Read the model definition and answer for the solid it produces. Units are mm, in the model's axes. A direction names the side the tool comes from. Round coordinates to 2 decimals unless told otherwise and drop trailing zeros. Order: outer loops, then holes, each group sorted by start corner. A loop starts at its lowest first (then second) coordinate and runs counter-clockwise, first axis right, second up. Notation, with made-up numbers: (2.25, -27) -> (17.25, -27) arc R29 ccw to (17.25, 5) -> close; hole circle Ø11 at (-19, 11). An arc over 180 degrees is marked (long way). One line per item, written item: value. Start each with the question number.
1. Section D-D (z = -27) is taken. Give the vertices of the cut face in (x, y), then the cut area to 3 significant figures.
2. The mould has two halves that part along Z. Classify faces 3 (the face through (44.014, 2.465, -24.759)), 4 (the face through (-0.565, 2.465, 50.497)), 5 (the face through (0, 3, -6)): released by +Z, released by -Z, zero draft, split by the parting line, or undercut.
3. Section A-A (x = 0) is taken. Give the vertices of the cut face in (y, z) (3 decimals).
4. Flat-ended cylindrical pins translate along their axes: pin 1 Ø1.5 at (x, z) = (28, 16) entering from -Y; pin 2 Ø1 at (x, y) = (-7, 3) entering from +Z; pin 3 Ø1.5 at (x, y) = (-1, 2.5) entering from +Z. Find the tip coordinate at first contact, or state that the pin passes through.
5. For faces 1 (the face through (-30.64, 2.54, 34.6)), 2 (the face through (39.43, 2.535, 22.706)), determine the directions among +Z, -Z, +X, -X, +Y, -Y from which every point of the face is accessible in a straight line to the end or side of a thin tool.
6. Consider line 1 (X direction, y = 4.8, z = 17.5); line 2 (X direction, y = 2.4, z = -4); line 3 (X direction, y = 3.2, z = -39.75). Determine where each line is inside the solid, lowest interval first.
7. Section C-C (z = -39.75) is taken. Give the vertices of the cut face in (x, y), then the cut area to 3 significant figures.
8. Section B-B (z = -16) is taken. Give the vertices of the cut face in (x, y).
from build123d import *

# Parameters (mm, degrees)
SKETCH1_R                = 50.5
SKETCH1_R_2              = 5.675
BOSS_EXTRUDE1_DEPTH      = 5
SKETCH4_R                = 1.7
CUT_EXTRUDE5_DEPTH       = 72.592597383
SKETCH8_R                = 1.7
CUT_EXTRUDE9_DEPTH       = 72.592597383
SKETCH9_R                = 1.7
CUT_EXTRUDE10_DEPTH      = 72.592597383
CIRPATTERN3_COUNT        = 3
CUT_EXTRUDE11_DEPTH      = 72.592597383
CIRPATTERN4_COUNT        = 3
SKETCH11_W               = 12
SKETCH11_H               = 12
CUT_EXTRUDE12_DEPTH      = 72.592597383
FILLET1_R                = 2
CUT_EXTRUDE13_DEPTH      = 72.592597383
FILLET2_R                = 10
CIRPATTERN5_COUNT        = 3
FILLET2_OF_CIRPATTERN5_R = 10


with BuildPart() as part:
    # Sketch1 → Boss-Extrude1 (new body)
    with BuildSketch(Plane(origin=(0, 0, 0), x_dir=(1, 0, 0), z_dir=(0, 1, 0))):
        with Locations(Location((0, 0, 0), (0, 0, 270))):
            Circle(SKETCH1_R)
        with Locations(Location((0, 28, 0), (0, 0, 270))):
            Circle(SKETCH1_R_2, mode=Mode.SUBTRACT)
        with Locations(Location((24.248711306, -14, 0), (0, 0, 270))):
            Circle(SKETCH1_R_2, mode=Mode.SUBTRACT)
        with Locations(Location((-24.248711306, -14, 0), (0, 0, 270))):
            Circle(SKETCH1_R_2, mode=Mode.SUBTRACT)
    extrude(amount=BOSS_EXTRUDE1_DEPTH)

    # Sketch4 → Cut-Extrude5 (cut, through all)
    with BuildSketch(Plane(origin=(0, 0, 0), x_dir=(1, 0, 0), z_dir=(0, 1, 0))):
        with Locations(Location((27.712812921, 16, 0), (0, 0, 270))):
            Circle(SKETCH4_R)
        with Locations(Location((0, -32, 0), (0, 0, 270))):
            Circle(SKETCH4_R)
        with Locations(Location((-27.712812921, 16, 0), (0, 0, 270))):
            Circle(SKETCH4_R)
    extrude(amount=CUT_EXTRUDE5_DEPTH, mode=Mode.SUBTRACT)

    # Sketch8 → Cut-Extrude9 (cut, through all)
    with BuildSketch(Plane(origin=(0, 5, 0), x_dir=(1, 0, 0), z_dir=(0, 1, 0))):
        with Locations(Location((11, 39.75, 0), (0, 0, 270))):
            Circle(SKETCH8_R)
        with Locations(Location((11, 15.75, 0), (0, 0, 270))):
            Circle(SKETCH8_R)
        with Locations(Location((-11, 39.75, 0), (0, 0, 90))):
            Circle(SKETCH8_R)
        with Locations(Location((-11, 15.75, 0), (0, 0, 90))):
            Circle(SKETCH8_R)
    cut_extrude9 = extrude(amount=-CUT_EXTRUDE9_DEPTH, mode=Mode.SUBTRACT)

    # Sketch9 → Cut-Extrude10 (cut, through all)
    with BuildSketch(Plane.XZ):
        with Locations(Location((-17.892304845, 39, 0), (0, 0, 270))):
            Circle(SKETCH9_R)
        with Locations(Location((17.892304845, 39, 0), (0, 0, 90))):
            Circle(SKETCH9_R)
    cut_extrude10 = extrude(amount=-CUT_EXTRUDE10_DEPTH, mode=Mode.SUBTRACT)

    # CirPattern3: Cut-Extrude9, Cut-Extrude10 ×3 about axis
    cirpattern3_axis = Axis((0, 0, 0), (0, 1, 0))
    add([cut_extrude9.rotate(cirpattern3_axis, i * 360 / CIRPATTERN3_COUNT) for i in range(1, CIRPATTERN3_COUNT)], mode=Mode.SUBTRACT)
    add([cut_extrude10.rotate(cirpattern3_axis, i * 360 / CIRPATTERN3_COUNT) for i in range(1, CIRPATTERN3_COUNT)], mode=Mode.SUBTRACT)

    # Sketch10 → Cut-Extrude11 (cut, through all)
    with BuildSketch(Plane(origin=(0, 5, 0), x_dir=(1, 0, 0), z_dir=(0, 1, 0))):
        with BuildLine():
            Line((-13.943212455, 41.732323521), (-15.36922282, 46.000402062))
            ThreePointArc((-15.36922282, 46.000402062), (-20.496985694, 43.955927671), (-25.359206382, 41.341996223))
            Line((-25.359206382, 41.341996223), (-23.006290326, 37.506140903))
            ThreePointArc((-23.006290326, 37.506140903), (-18.595203517, 39.87754263), (-13.943212455, 41.732323521))
        make_face()
    cut_extrude11 = extrude(amount=-CUT_EXTRUDE11_DEPTH, mode=Mode.SUBTRACT)

    # CirPattern4: Cut-Extrude11 ×3 about axis
    cirpattern4_axis = Axis((0, 0, 0), (0, 1, 0))
    for i in range(1, CIRPATTERN4_COUNT):
        add(cut_extrude11.rotate(cirpattern4_axis, i * 360 / CIRPATTERN4_COUNT), mode=Mode.SUBTRACT)

    # Sketch11 → Cut-Extrude12 (cut, through all)
    with BuildSketch(Plane(origin=(0, 5, 0), x_dir=(1, 0, 0), z_dir=(0, 1, 0))):
        Rectangle(SKETCH11_W, SKETCH11_H)
    extrude(amount=-CUT_EXTRUDE12_DEPTH, mode=Mode.SUBTRACT)

    # Fillet1
    fillet1_edges = [part.edges().sort_by_distance(p)[0] for p in [
        (6, 2.5, -6),
        (6, 2.5, 6),
        (-6, 2.5, 6),
        (-6, 2.5, -6),
    ]]
    fillet(fillet1_edges, radius=FILLET1_R)

    # Sketch12 → Cut-Extrude13 (cut, through all)
    with BuildSketch(Plane(origin=(0, 5, 0), x_dir=(1, 0, 0), z_dir=(0, 1, 0))):
        with BuildLine():
            ThreePointArc((46.016854863, -20.801419868), (39.404155872, -22.75), (41.022985472, -29.45105538))
            ThreePointArc((41.022985472, -29.45105538), (43.734282891, -25.25), (46.016854863, -20.801419868))
        make_face()
    cut_extrude13 = extrude(amount=-CUT_EXTRUDE13_DEPTH, mode=Mode.SUBTRACT)

    # Fillet2
    fillet2_edges = [part.edges().sort_by_distance(p)[0] for p in [
        (46.016854863, 2.5, 20.801419868),
        (41.022985472, 2.5, 29.45105538),
    ]]
    fillet(fillet2_edges, radius=FILLET2_R)

    # CirPattern5: Cut-Extrude13 ×3 about axis
    cirpattern5_axis = Axis((0, 0, 0), (0, 1, 0))
    for i in range(1, CIRPATTERN5_COUNT):
        add(cut_extrude13.rotate(cirpattern5_axis, i * 360 / CIRPATTERN5_COUNT), mode=Mode.SUBTRACT)

    # Fillet2 of CirPattern5
    fillet2_of_cirpattern5_edges = [part.edges().sort_by_distance(p)[0] for p in [
        (-4.993869391, 2.5, -50.252475248),
        (4.993869391, 2.5, -50.252475248),
        (-41.022985472, 2.5, 29.45105538),
        (-46.016854863, 2.5, 20.801419868),
    ]]
    fillet(fillet2_of_cirpattern5_edges, radius=FILLET2_OF_CIRPATTERN5_R)


solid = part.part
Answer:
1. outline: (-42.68, 0) -> (-5.59, 0) -> (-5.59, 5) -> (-42.68, 5) -> close; (5.59, 0) -> (42.68, 0) -> (42.68, 5) -> (5.59, 5) -> close
1. area: 371 mm^2
2. face 3: split by the parting line
2. face 4: released by +Z
2. face 5: undercut
3. outline: (0, -45.5) -> (5, -45.5) -> (5, -33.675) -> (0, -33.675) -> close; (0, -22.325) -> (5, -22.325) -> (5, -6) -> (0, -6) -> close; (0, 6) -> (5, 6) -> (5, 30.3) -> (0, 30.3) -> close; (0, 33.7) -> (5, 33.7) -> (5, 50.5) -> (0, 50.5) -> close
4. pin 1: through
4. pin 2: z = 50.08
4. pin 3: z = 50.5
5. face 1: +Y, -Y
5. face 2: +X, +Y, -Y
6. line 1: -46.59 to -28.72, -19.78 to -9.84, -6.44 to 6.44, 9.84 to 19.78, 28.72 to 46.59
6. line 2: -50.34 to -44.42, -41.02 to -6, 6 to 41.02, 44.42 to 50.34
6. line 3: -31.15 to -24.38, -18.87 to -12.7, -9.3 to 9.3, 12.7 to 31.15
7. outline: (-31.15, 0) -> (-24.38, 0) -> (-24.38, 5) -> (-31.15, 5) -> close; (-18.87, 0) -> (-12.7, 0) -> (-12.7, 5) -> (-18.87, 5) -> close; (-9.3, 0) -> (9.3, 0) -> (9.3, 5) -> (-9.3, 5) -> close; (12.7, 0) -> (31.15, 0) -> (31.15, 5) -> (12.7, 5) -> close
7. area: 250 mm^2
8. outline: (-47.9, 0) -> (-29.41, 0) -> (-29.41, 5) -> (-47.9, 5) -> close; (-26.01, 0) -> (-12.68, 0) -> (-12.68, 5) -> (-26.01, 5) -> close; (-9.32, 0) -> (9.32, 0) -> (9.32, 5) -> (-9.32, 5) -> close; (12.68, 0) -> (26.01, 0) -> (26.01, 5) -> (12.68, 5) -> close; (29.41, 0) -> (47.9, 0) -> (47.9, 5) -> (29.41, 5) -> close
